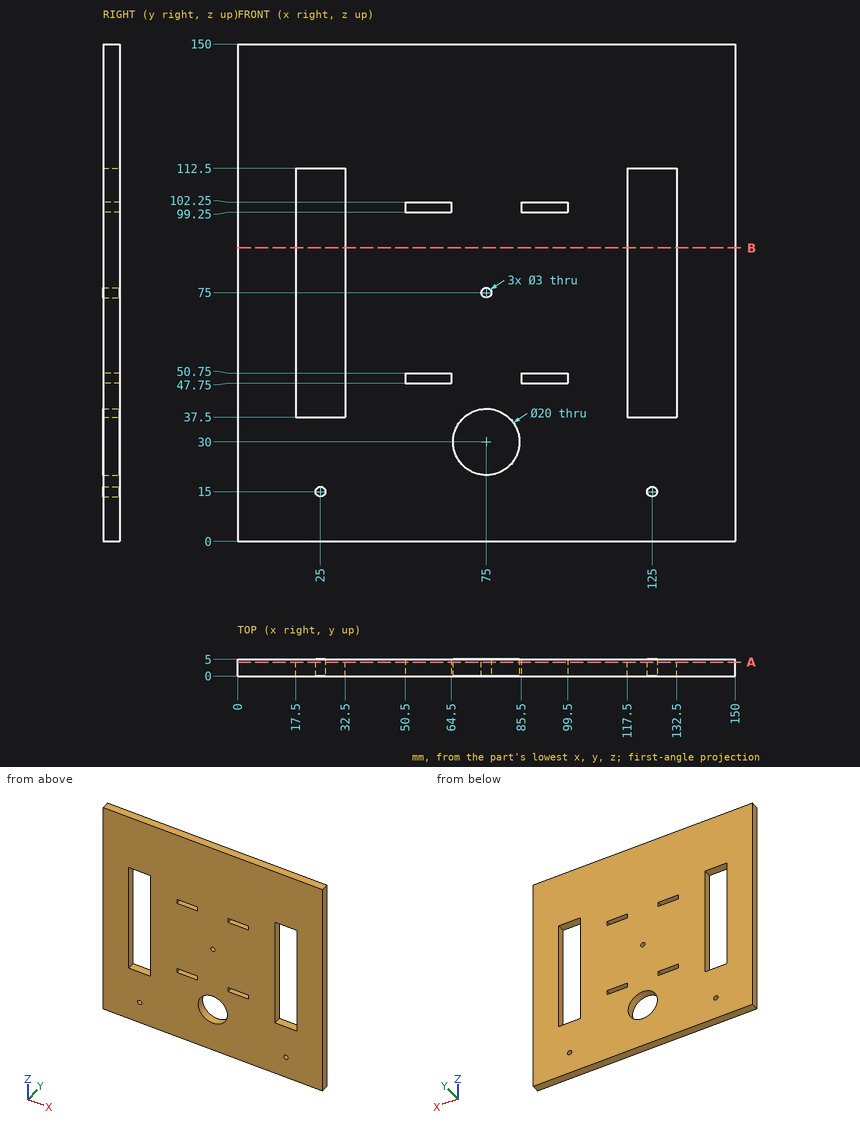
Geometry: see drawing. Coordinates: mm, zero at the bounding-box minimum. Round coordinates to 2 decimals unless told otherwise and drop trailing zeros. Loops run counter-clockwise (first coordinate to the right, second up) from the corner with the lowest first, then second, coordinate; pieces in that order, holes last. Notation, with made-up numbers: (76.5, -39.75) - (97.5, -39.75) arc R21 ccw to (97.5, -11.75) - close; hole circle Ø4 at (-20, 29). An arc over 180 degrees is marked (long way). Write item = value, one per line. Start each with the question number.
(1) Ray query, line 1 along Z through (x, y) = (95, 0.55); line 2 along X through (y, z) = (3.25, 75); line 3 along X through (y, z) = (1.75, 101.5). Return the intervals inside material, ascending. Write a range as from..to.
(2) Section query A-A, the plane y = 4.2. State how many separate pieces and enclosed holes the cut face has, plus the area to 3 significant figures.
(3) Section query B-B, the plane z = 88.5. Output: boundary loops of the cut face in (x, y).
Conclusion:
q1.line_1 = 0..47.75, 50.75..99.25, 102.25..150
q1.line_2 = 0..17.5, 32.5..73.5, 76.5..117.5, 132.5..150
q1.line_3 = 0..17.5, 32.5..50.5, 64.5..85.5, 99.5..117.5, 132.5..150
q2.separate_pieces = 1
q2.enclosed_holes = 10
q2.area = 19,700 mm2
q3.outline = (0, 0) - (17.5, 0) - (17.5, 5) - (0, 5) - close; (32.5, 0) - (117.5, 0) - (117.5, 5) - (32.5, 5) - close; (132.5, 0) - (150, 0) - (150, 5) - (132.5, 5) - close
